Check sheet for the modelled part. Datum: model origin and axes. Units: mm. A direction names the side the tool comes from. Round coordinates to 2 decimals unless told otherwise and drop trailing zeros. Write each loop counter-clockwise with the first axis right and the second up, starting at its lowest first coordinate (ties: lowest second). Pieces come first, ordered by that corner, then holes. Notation, with made-up numbers: (39.5, 85.25) -> (45.5, 85.25) arc R28 cw to (45.5, 117.25) -> close; hole circle Ø4 at (86, 81). An arc over 180 degrees is marked (long way). Write item = value, one per line.
from build123d import *

# Parameters (mm, degrees)
BOSS_EXTRUDE1_DEPTH = 55
BOSS_EXTRUDE2_START = 2
BOSS_EXTRUDE2_DEPTH = 2
BOSS_EXTRUDE3_START = 2
BOSS_EXTRUDE3_DEPTH = 2
BOSS_EXTRUDE5_START = 2
BOSS_EXTRUDE5_DEPTH = 2
BOSS_EXTRUDE6_DEPTH = 2
SKETCH7_W           = 3.4
SKETCH7_H           = 11.3
CUT_EXTRUDE2_DEPTH  = 55
SKETCH8_R           = 2.15
CUT_EXTRUDE3_DEPTH  = 6
SKETCH9_R           = 2.7
CUT_EXTRUDE4_DEPTH  = 12.6
LPATTERN1_COUNT     = 2
LPATTERN1_PITCH     = 37
LPATTERN2_COUNT     = 2
LPATTERN2_PITCH     = 41
FILLET1_R           = 3


with BuildPart() as part:
    # Sketch1 → Boss-Extrude1 (new body)
    with BuildSketch(Plane.XY):
        with BuildLine():
            Line((0, 0), (0, -93.2))
            Line((0, -93.2), (-6, -93.2))
            Line((-6, -93.2), (-6, -81.2))
            Line((-6, -81.2), (-16, -81.2))
            Line((-16, -81.2), (-16, -74.2))
            ThreePointArc((-16, -74.2), (-8.4, -66.6), (-16, -59))
            Line((-16, -59), (-16, -44.3))
            Line((-16, -44.3), (-10.5, -44.3))
            Line((-10.5, -44.3), (-10.5, -37.6))
            Line((-10.5, -37.6), (-16, -37.6))
            Line((-16, -37.6), (-16, -34.2))
            ThreePointArc((-16, -34.2), (-8.4, -26.6), (-16, -19))
            Line((-16, -19), (-16, -12))
            Line((-16, -12), (-6, -12))
            Line((-6, -12), (-6, 0))
            Line((-6, 0), (0, 0))
        make_face()
    extrude(amount=BOSS_EXTRUDE1_DEPTH)

    # Sketch2 → Boss-Extrude2 (add)
    with BuildSketch(Plane(origin=(0, 0, 28.5), x_dir=(-1, 0, 0), z_dir=(0, 0, -1)).offset(BOSS_EXTRUDE2_START)):
        with BuildLine():
            Line((16, -34.2), (16, -31.5))
            ThreePointArc((16, -31.5), (11.1, -26.6), (16, -21.7))
            Line((16, -21.7), (16, -19))
            ThreePointArc((16, -19), (8.4, -26.6), (16, -34.2))
        make_face()
    extrude(amount=-BOSS_EXTRUDE2_DEPTH)

    # Sketch3 → Boss-Extrude3 (add)
    with BuildSketch(Plane(origin=(0, 0, 28.5), x_dir=(-1, 0, 0), z_dir=(0, 0, -1)).offset(BOSS_EXTRUDE3_START)):
        with BuildLine():
            Line((16, -74.2), (16, -71.5))
            ThreePointArc((16, -71.5), (11.1, -66.6), (16, -61.7))
            Line((16, -61.7), (16, -59))
            ThreePointArc((16, -59), (8.4, -66.6), (16, -74.2))
        make_face()
    extrude(amount=-BOSS_EXTRUDE3_DEPTH)

    # Sketch4 → Boss-Extrude5 (add)
    with BuildSketch(Plane(origin=(0, 0, 2), x_dir=(-1, 0, 0), z_dir=(0, 0, -1)).offset(BOSS_EXTRUDE5_START)):
        with BuildLine():
            Line((16, -59), (16, -61.7))
            ThreePointArc((16, -61.7), (11.1, -66.6), (16, -71.5))
            Line((16, -71.5), (16, -74.2))
            ThreePointArc((16, -74.2), (8.4, -66.6), (16, -59))
        make_face()
        with BuildLine():
            Line((16, -19), (16, -21.7))
            ThreePointArc((16, -21.7), (11.1, -26.6), (16, -31.5))
            Line((16, -31.5), (16, -34.2))
            ThreePointArc((16, -34.2), (8.4, -26.6), (16, -19))
        make_face()
    extrude(amount=-BOSS_EXTRUDE5_DEPTH)

    # Sketch5 → Boss-Extrude6 (add)
    with BuildSketch(Plane(origin=(0, 0, 53), x_dir=(-1, 0, 0), z_dir=(0, 0, -1))):
        with BuildLine():
            Line((16, -19), (16, -21.7))
            ThreePointArc((16, -21.7), (11.1, -26.6), (16, -31.5))
            Line((16, -31.5), (16, -34.2))
            ThreePointArc((16, -34.2), (8.4, -26.6), (16, -19))
        make_face()
        with BuildLine():
            Line((16, -59), (16, -61.7))
            ThreePointArc((16, -61.7), (11.1, -66.6), (16, -71.5))
            Line((16, -71.5), (16, -74.2))
            ThreePointArc((16, -74.2), (8.4, -66.6), (16, -59))
        make_face()
    extrude(amount=-BOSS_EXTRUDE6_DEPTH)

    # Sketch7 → Cut-Extrude2 (cut)
    with BuildSketch(Plane.XY.offset(55)):
        with Locations((-14.3, -49.95)):
            Rectangle(SKETCH7_W, SKETCH7_H)
    extrude(amount=-CUT_EXTRUDE2_DEPTH, mode=Mode.SUBTRACT)

    # Sketch8 → Cut-Extrude3 (cut)
    with BuildSketch(Plane(origin=(0, 0, 0), x_dir=(0, 0, -1), z_dir=(1, 0, 0))):
        with Locations(Location((-46, -6, 0), (0, 0, 90))):
            Circle(SKETCH8_R)
        with Locations(Location((-9, -6, 0), (0, 0, 90))):
            Circle(SKETCH8_R)
        with Locations(Location((-7, -87.2, 0), (0, 0, 90))):
            Circle(SKETCH8_R)
        with Locations(Location((-48, -87.2, 0), (0, 0, 90))):
            Circle(SKETCH8_R)
    extrude(amount=-CUT_EXTRUDE3_DEPTH, mode=Mode.SUBTRACT)

    # Sketch9 → Cut-Extrude4 (cut)
    with BuildSketch(Plane(origin=(0, 0, 0), x_dir=(0, 0, -1), z_dir=(1, 0, 0))):
        with Locations(Location((-27.5, -48.6, 0), (0, 0, 90))):
            Circle(SKETCH9_R)
    extrude(amount=-CUT_EXTRUDE4_DEPTH, mode=Mode.SUBTRACT)

    # Cut-Loft1: read off the stored shape, not the designer's step
    # Cut-Loft1: loft between two sections, ruled curve by curve
    cut_loft1_from = [
        Edge.make_bspline([(0, -9.090752309, 49.270665095), (0, -2.54942212, 55.452169714), (0, 3.632082499, 48.910839524), (0, -2.909247691, 42.729334905), (0, -9.45057788, 36.547830286), (0, -15.632082499, 43.089160476), (0, -9.090752309, 49.270665095)], [0, 0, 0, 0, 0.5, 0.5, 0.5, 1, 1, 1, 1], 3, [1, 0.333333333, 0.333333333, 1, 0.333333333, 0.333333333, 1]),
    ]
    cut_loft1_to = [
        Edge.make_bspline([(-2.5, -7.797727139, 47.179269746), (-2.5, -5.439187646, 50.774724024), (-2.5, -1.843733369, 48.416184531), (-2.5, -4.202272861, 44.820730254), (-2.5, -6.560812354, 41.225275976), (-2.5, -10.156266631, 43.583815469), (-2.5, -7.797727139, 47.179269746)], [0, 0, 0, 0, 0.5, 0.5, 0.5, 1, 1, 1, 1], 3, [1, 0.333333333, 0.333333333, 1, 0.333333333, 0.333333333, 1]),
    ]
    cut_loft1 = Solid(Shell([*[Face.make_surface_from_curves(cut_loft1_from[k], cut_loft1_to[k]) for k in range(1)], Face(Wire(cut_loft1_from)), Face(Wire(cut_loft1_to))]))
    add(cut_loft1, mode=Mode.SUBTRACT)

    # LPattern1: Cut-Loft1 ×2
    with Locations(*[(0, 0, -i * LPATTERN1_PITCH) for i in range(1, LPATTERN1_COUNT)]):
        add(cut_loft1, mode=Mode.SUBTRACT)

    # Cut-Loft2: read off the stored shape, not the designer's step
    # Cut-Loft2: loft between two sections, ruled curve by curve
    cut_loft2_from = [
        Edge.make_bspline([(-2.5, -88.803773463, 46.568074485), (-2.5, -85.939922433, 43.36052756), (-2.5, -82.732375507, 46.22437859), (-2.5, -85.596226537, 49.431925515), (-2.5, -88.460077567, 52.63947244), (-2.5, -91.667624493, 49.77562141), (-2.5, -88.803773463, 46.568074485)], [0, 0, 0, 0, 0.5, 0.5, 0.5, 1, 1, 1, 1], 3, [1, 0.333333333, 0.333333333, 1, 0.333333333, 0.333333333, 1]),
    ]
    cut_loft2_to = [
        Edge.make_bspline([(0, -88.245004687, 43.623018711), (0, -79.491042109, 41.533009337), (0, -77.401032735, 50.286971915), (0, -86.154995313, 52.376981289), (0, -94.908957891, 54.466990663), (0, -96.998967265, 45.713028085), (0, -88.245004687, 43.623018711)], [0, 0, 0, 0, 0.5, 0.5, 0.5, 1, 1, 1, 1], 3, [1, 0.333333333, 0.333333333, 1, 0.333333333, 0.333333333, 1]),
    ]
    cut_loft2 = Solid(Shell([*[Face.make_surface_from_curves(cut_loft2_from[k], cut_loft2_to[k]) for k in range(1)], Face(Wire(cut_loft2_from)), Face(Wire(cut_loft2_to))]))
    add(cut_loft2, mode=Mode.SUBTRACT)

    # LPattern2: Cut-Loft2 ×2
    with Locations(*[(0, 0, -i * LPATTERN2_PITCH) for i in range(1, LPATTERN2_COUNT)]):
        add(cut_loft2, mode=Mode.SUBTRACT)

    # Fillet1
    # the kernel refuses this fillet: 3 mm, written as the material it takes off along each edge
    with BuildSketch(Plane(origin=(0, 7.5, 0), x_dir=(-1, 0, 0), z_dir=(0, -1, 0))) as fillet1_piece_1:
        with BuildLine():
            CenterArc((FILLET1_R, -FILLET1_R), FILLET1_R, 90, 90)
            Line((0, -FILLET1_R), (0, 0))
            Line((0, 0), (FILLET1_R, 0))
        make_face()
    extrude(amount=108.2, mode=Mode.SUBTRACT)
    with BuildSketch(Plane(origin=(0, 7.5, 55), x_dir=(-1, 0, 0), z_dir=(0, -1, 0))) as fillet1_piece_2:
        with BuildLine():
            CenterArc((FILLET1_R, FILLET1_R), FILLET1_R, 180, 90)
            Line((0, FILLET1_R), (0, 0))
            Line((0, 0), (FILLET1_R, 0))
        make_face()
    extrude(amount=108.2, mode=Mode.SUBTRACT)


solid = part.part
(1) Release check for a two-part mould opening along Z. For faces 4 (the flat face through (-16, -77, 27)), 5 (the flat face through (-8, -46, 0)), 6 (the cylindrical face through (-6.212, -46.025, 28.311)) record: pulls with the +Z half, pulls with the -Z half, needs draft (parallel to the pull), parting line crosses it, or undercut.
Worked answers:
face_4 = needs draft
face_5 = pulls with the -Z half
face_6 = undercut
(2) Access from +Z, -Z, +X, -X, +Y, -Y to the whole of each face (thin tool, end or side, straight path). Record for faces 1 (the flat face through (-10, -66, 28.5)), 2 (the flat face through (-12.6, -53, 28)), 3 (the cylindrical face through (-4.23, -4.84, 47.81)).
Worked answers:
face_1 = -X
face_2 = +Z, -Z, -X
face_3 = +X, -X
(3) Sectioned sample at D-D on y = -87.2. Count the separate pieces of the cut face and the enclosed holes in it, then the cut area to 3 significant figures.
Worked answers:
separate_pieces = 3
enclosed_holes = 0
area = 264 mm²
(4) Sectioned sample at C-C on y = -26.6. Enter the section's corners in (x, z).
Worked answers:
outline = (-11.1, 0) -> (-3, 0) arc R3 ccw to (0, 3) -> (0, 52) arc R3 ccw to (-3, 55) -> (-11.1, 55) -> (-11.1, 53) -> (-8.4, 53) -> (-8.4, 28.5) -> (-11.1, 28.5) -> (-11.1, 26.5) -> (-8.4, 26.5) -> (-8.4, 2) -> (-11.1, 2) -> close
(5) Go/stop test with flat-tipped pins: P1, Ø3.5, axis at x = -13.5, z = 35.5, coming from the +Y side; P2, Ø5.5, axis at y = -48.5, z = 15, coming from the -X side; P3, Ø5, axis at y = -6, z = 9, coming from the +X side; P4, Ø3.5, axis at y = -87.2, z = 7, coming from the +X side. Record where each tip stops, or that it passes through.
Worked answers:
P1 = -12
P2 = -12.6
P3 = -2.11
P4 = through
(6) Sectioned sample at A-A on y = -48.6. Enter the section's corners in (x, z), then the cut area to 3 significant figures.
Worked answers:
outline = (-12.6, 0) -> (-3, 0) arc R3 ccw to (0, 3) -> (0, 24.8) -> (-12.6, 24.8) -> close; (-12.6, 30.2) -> (0, 30.2) -> (0, 52) arc R3 ccw to (-3, 55) -> (-12.6, 55) -> close
area = 621 mm²
(7) Sectioned sample at B-B on z = 27.5. Enter the section's corners in (x, y).
Worked answers:
outline = (-16, -81.2) -> (-6, -81.2) -> (-6, -93.2) -> (0, -93.2) -> (0, -51.3) -> (-12.6, -51.3) -> (-12.6, -55.6) -> (-16, -55.6) -> (-16, -61.7) arc R4.9 cw to (-16, -71.5) -> close; (-16, -37.6) -> (-10.5, -37.6) -> (-10.5, -44.3) -> (-12.6, -44.3) -> (-12.6, -45.9) -> (0, -45.9) -> (0, 0) -> (-6, 0) -> (-6, -12) -> (-16, -12) -> (-16, -21.7) arc R4.9 cw to (-16, -31.5) -> close
(8) Material ranges on L1, parallel to Z at x = -3.8, y = -87.2; L2, parallel to Z at x = -3.4, y = -6; L3, parallel to Z at x = -4.75, y = -48.6, recorded low to high. Write a range as [from, to].
Worked answers:
L1 = [0, 4.85], [9.15, 45.85], [50.15, 55]
L2 = [0, 6.85], [11.15, 43.85], [48.15, 55]
L3 = [0, 24.8], [30.2, 55]
